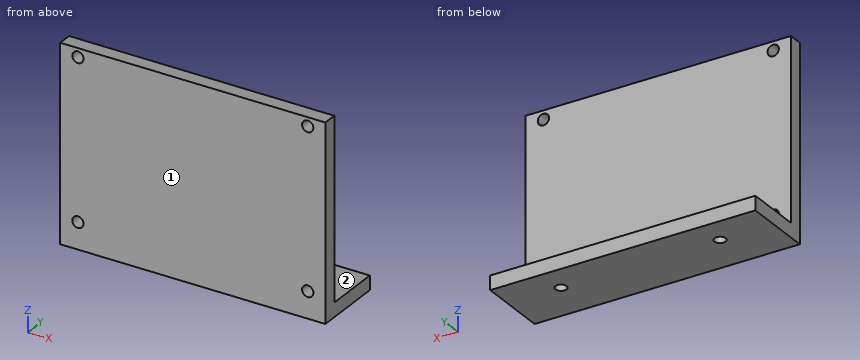
```python
from build123d import *

# Parameters (mm, degrees)
SKETCH1_W           = 75
SKETCH1_H           = 55
BOSS_EXTRUDE1_DEPTH = 20
SKETCH2_W           = 51
SKETCH2_H           = 16
CUT_EXTRUDE1_DEPTH  = 94
SKETCH3_R           = 1.6
CUT_EXTRUDE2_DEPTH  = 54
SKETCH4_R           = 1.6
CUT_EXTRUDE3_DEPTH  = 10


with BuildPart() as part:
    # Sketch1 → Boss-Extrude1 (new body)
    with BuildSketch(Plane(origin=(0, 0, 0), x_dir=(1, 0, 0), z_dir=(0, 1, 0))):
        with Locations((37.5, 27.5)):
            Rectangle(SKETCH1_W, SKETCH1_H)
    extrude(amount=BOSS_EXTRUDE1_DEPTH)

    # Sketch2 → Cut-Extrude1 (cut)
    with BuildSketch(Plane(origin=(75, 0, 0), x_dir=(0, 0, -1), z_dir=(1, 0, 0))):
        with Locations((25.5, 12)):
            Rectangle(SKETCH2_W, SKETCH2_H)
    extrude(amount=-CUT_EXTRUDE1_DEPTH, mode=Mode.SUBTRACT)

    # Sketch3 → Cut-Extrude2 (cut)
    with BuildSketch(Plane(origin=(0, 0, -55), x_dir=(-1, 0, 0), z_dir=(0, 0, -1))):
        with Locations((-60, 12)):
            Circle(SKETCH3_R)
        with Locations((-15, 12)):
            Circle(SKETCH3_R)
    extrude(amount=-CUT_EXTRUDE2_DEPTH, mode=Mode.SUBTRACT)

    # Sketch4 → Cut-Extrude3 (cut)
    with BuildSketch(Plane.XZ):
        with Locations((5, -2.5)):
            Circle(SKETCH4_R)
        with Locations((5, -47.5)):
            Circle(SKETCH4_R)
        with Locations((70, -47.5)):
            Circle(SKETCH4_R)
        with Locations((70, -2.5)):
            Circle(SKETCH4_R)
    extrude(amount=-CUT_EXTRUDE3_DEPTH, mode=Mode.SUBTRACT)


solid = part.part
```
Read the model definition and answer for the solid it produces. Units are mm, in the model's axes. Face numbers are marked on the shaded views. A direction names the side the tool comes from. Give positions to 0.01 mm unless a question says otherwise; leave off trailing zeros. Order: outer loops, then holes, each group sorted by start corner. A loop starts at its lowest first (then second) coordinate and runs counter-clockwise, first axis right, second up. Notation, with made-up numbers: (73, 6) -> (107, 6) arc R30 ccw to (107, 42) -> close; hole circle Ø11 at (-6.5, -35.5). An arc over 180 degrees is marked (long way). One line per item, written item: value. Start each with the question number.
(1) Straight lines are drawn through the part: L1, parallel to Z at x = 70, y = 1.1; L2, parallel to Y at x = 18.5, z = -12; L3, parallel to Y at x = 15, z = -53. For each, find the intervals that lie inside material, in ascending order.
(2) Flat-ended cylindrical pins translate along their axes: P1, Ø3, axis at x = 17.5, z = -40, coming from the +Y side; P2, Ø5, axis at x = 42.5, y = 13.5, coming from the +Z side; P3, Ø2.5, axis at x = 5, z = -2.5, coming from the -Y side. Find the tip coordinate at first contact, or state that the pin passes through.
(3) The part is cut by section C-C (x = 60). Determine the outline of the cut face in (y, z).
(4) The part is cut by section B-B (z = -2.5). Determine the outline of the cut face in (x, y).
(5) The part is cut by section A-A (x = 5). Determine the outline of the cut face in (y, z), and give its area (3 significant figures).
(6) The part is cut by section D-D (y = 12). Determine the outline of the cut face in (x, z), and give its area (3 significant figures).
(7) A tool of negligible diameter and unlimited length cuts with its end or side. For the marked faces 1 and 2, from which of +Z, -Z, +X, -X, +Y, -Y can it reach the whole face along a straight path? Write none if from no direction.
Taken from the geometry:
1. L1: -55 to -49.1, -45.9 to -4.1, -0.9 to 0
1. L2: 0 to 4
1. L3: 0 to 10.4, 13.6 to 20
2. P1: y = 4
2. P2: z = -51
2. P3: through
3. outline: (0, -55) -> (10.4, -55) -> (10.4, -51) -> (4, -51) -> (4, 0) -> (0, 0) -> close; (13.6, -55) -> (20, -55) -> (20, -51) -> (13.6, -51) -> close
4. outline: (0, 0) -> (3.4, 0) -> (3.4, 4) -> (0, 4) -> close; (6.6, 0) -> (68.4, 0) -> (68.4, 4) -> (6.6, 4) -> close; (71.6, 0) -> (75, 0) -> (75, 4) -> (71.6, 4) -> close
5. outline: (0, -55) -> (20, -55) -> (20, -51) -> (4, -51) -> (4, -49.1) -> (0, -49.1) -> close; (0, -45.9) -> (4, -45.9) -> (4, -4.1) -> (0, -4.1) -> close; (0, -0.9) -> (4, -0.9) -> (4, 0) -> (0, 0) -> close
5. area: 258 mm^2
6. outline: (0, -55) -> (13.4, -55) -> (13.4, -51) -> (0, -51) -> close; (16.6, -55) -> (58.4, -55) -> (58.4, -51) -> (16.6, -51) -> close; (61.6, -55) -> (75, -55) -> (75, -51) -> (61.6, -51) -> close
6. area: 274 mm^2
7. face 1: +Z, -Z, +X, -X, -Y
7. face 2: +Z, +X, -X, +Y
